Check sheet for the modelled part. Datum: model origin and axes. Units: mm. A direction names the side the tool comes from. Round coordinates to 2 decimals unless told otherwise and drop trailing zeros. Order: outer loops, then holes, each group sorted by start corner. A loop starts at its lowest first (then second) coordinate and runs counter-clockwise, first axis right, second up.
Q1. Scan lines: probe 1 along X at (y, z) = (-9, -7.5); probe 2 along Z at (x, y) = (69, 0); probe 3 along X at (y, z) = (-3.5, -5.5). Record each from-to range of solid material in increasing order.
Q2. Cross-section at A-A on x = -5. Record the cut outline in (y, z) (3 decimals), then the cut area to 3 significant figures.
Q3. Depth check by flat-ended pin: P1, Ø8.5, axis at x = -6.65, z = 0, coming from the +Y side (3 decimals); P2, Ø1.1, axis at y = 2, z = 13.5, coming from the -X side; P3, Ø1.5, axis at y = -4.5, z = -10.5, coming from the +X side; P4, Ø12, axis at y = 6, z = 7.5, coming from the +X side. Enter the tip coordinate at first touch or a pass-through.
Q4. Mould release check, pull along Y, two halves, no side actions. Record for faces 1 (the flat face through (70, 5.08, 7)), 2 (the cylindrical face through (68.61, 0.07, 10.11)), 3 (the cylindrical face through (61.14, 0.51, -12.69)): +Y half, -Y half, draft (parallel to the pull), parting line (faces both ways), or undercut.
Q5. Set-up check for faces 4 (the flat face through (33, 3.175, 10)), 5 (the cylindrical face through (70.05, -0.11, -5.08)), 6 (the flat face through (8, -3.175, 12.5)), 7 (the flat face through (33, 0, 10.16)): record each of +Z, -Z, +X, -X, +Y, -Y from which the full face is reachable in a straight line by a thin tool's end or side.
Q6. Cross-section at B-B on x = 57.5. Record the cut outline in (y, z) (3 decimals), then the cut area to 3 significant figures.
from build123d import *

# Parameters (mm, degrees)
F0_R     = 3.175
F2_DEPTH = 3.175
F3_R     = 1.524
F4_DEPTH = 7.62
F5_R     = 1.524
F6_DEPTH = 17.78
F7_R     = 1.524
F8_DEPTH = 10.414


with BuildPart() as f1:
    # F0 (on Front) → F1 (revolve)
    with BuildSketch(Plane.XZ):
        with BuildLine():
            Line((0, 15.238884), (0, 0))
            Line((0, 0), (7.112, 0))
            Line((7.112, 0), (66.294, 0))
            Line((66.294, 0), (66.294, 12.7))
            Line((66.294, 12.7), (56.134, 12.7))
            Line((56.134, 12.7), (56.134, 11.43))
            ThreePointArc((56.134, 11.43), (55.762026, 10.531974), (54.864, 10.16))
            Line((54.864, 10.16), (11.43, 10.16))
            ThreePointArc((11.43, 10.16), (10.531974, 10.531974), (10.16, 11.43))
            Line((10.16, 11.43), (10.16, 12.7))
            Line((10.16, 12.7), (7.112, 12.7))
            ThreePointArc((7.112, 12.7), (6.213974, 13.071974), (5.842, 13.97))
            Line((5.842, 13.97), (5.842, 15.24))
            Line((5.842, 15.24), (0.053232, 15.24))
            ThreePointArc((0.053232, 15.24), (0.02661, 15.239721), (0, 15.238884))
        make_face()
    revolve(axis=Axis((36.703, 0, 0), (-1, 0, 0)))

    # F0 (on Front) → F2 (join, symmetric)
    with BuildSketch(Plane.XZ):
        with BuildLine():
            Line((-0.9398, 0), (0, 0))
            Line((0, 0), (0, 15.238884))
            ThreePointArc((0, 15.238884), (-0.484346, 15.120613), (-0.885841, 14.82501))
            Line((-0.885841, 14.82501), (-10.88063, 3.847543))
            ThreePointArc((-10.88063, 3.847543), (-4.591961, 5.329721), (-0.9398, 0))
        make_face()
        with BuildLine():
            Line((0, 15.238884), (0, 0))
            Line((0, 0), (7.112, 0))
            Line((7.112, 0), (66.294, 0))
            Line((66.294, 0), (66.294, 12.7))
            Line((66.294, 12.7), (56.134, 12.7))
            Line((56.134, 12.7), (56.134, 11.43))
            ThreePointArc((56.134, 11.43), (55.762026, 10.531974), (54.864, 10.16))
            Line((54.864, 10.16), (11.43, 10.16))
            ThreePointArc((11.43, 10.16), (10.531974, 10.531974), (10.16, 11.43))
            Line((10.16, 11.43), (10.16, 12.7))
            Line((10.16, 12.7), (7.112, 12.7))
            ThreePointArc((7.112, 12.7), (6.213974, 13.071974), (5.842, 13.97))
            Line((5.842, 13.97), (5.842, 15.24))
            Line((5.842, 15.24), (0.053232, 15.24))
            ThreePointArc((0.053232, 15.24), (0.02661, 15.239721), (0, 15.238884))
        make_face()
        with BuildLine():
            Line((7.112, 0), (0, 0))
            Line((0, 0), (-0.9398, 0))
            ThreePointArc((-0.9398, 0), (-3.195791, -4.549339), (-8.182663, -5.506983))
            Line((-8.182663, -5.506983), (4.232475, -8.951452))
            ThreePointArc((4.232475, -8.951452), (5.340669, -8.738642), (5.842, -7.727678))
            Line((5.842, -7.727678), (5.842, -1.27))
            ThreePointArc((5.842, -1.27), (6.213974, -0.371974), (7.112, 0))
        make_face()
        with BuildLine():
            ThreePointArc((-8.182663, -5.506983), (-3.195791, -4.549339), (-0.9398, 0))
            ThreePointArc((-0.9398, 0), (-4.591961, 5.329721), (-10.88063, 3.847543))
            ThreePointArc((-10.88063, 3.847543), (-12.145978, -1.583727), (-8.182663, -5.506983))
        make_face()
        with Locations((-6.6548, 0)):
            Circle(F0_R, mode=Mode.SUBTRACT)
    extrude(amount=F2_DEPTH, both=True)

    # F3 (on face) → F4 (join)
    with BuildSketch(Plane.YZ.offset(66.294)):
        with BuildLine():
            ThreePointArc((-5.08, 0), (0, -5.08), (5.08, 0))
            ThreePointArc((5.08, 0), (0, 5.08), (-5.08, 0))
        make_face()
        Circle(F3_R, mode=Mode.SUBTRACT)
        with BuildLine():
            ThreePointArc((-5.08, 0), (0, 5.08), (5.08, 0))
            Line((5.08, 0), (5.08, 13.97))
            ThreePointArc((5.08, 13.97), (4.708026, 14.868026), (3.81, 15.24))
            Line((3.81, 15.24), (-3.81, 15.24))
            ThreePointArc((-3.81, 15.24), (-4.708026, 14.868026), (-5.08, 13.97))
            Line((-5.08, 13.97), (-5.08, 0))
        make_face()
    extrude(amount=F4_DEPTH)

    # F5 (on face) → F6 (cut)
    with BuildSketch(Plane.XY.offset(15.24)):
        with Locations((2.65662, 0)):
            Circle(F5_R)
    extrude(amount=-F6_DEPTH, mode=Mode.SUBTRACT)

    # F7 (on face) → F8 (cut)
    with BuildSketch(Plane.XY.offset(15.24)):
        with Locations((70.133381, 0)):
            Circle(F7_R)
    extrude(amount=-F8_DEPTH, mode=Mode.SUBTRACT)


solid = f1.part
Results found:
1. probe 1: x = 0 to 10.16, 56.13 to 66.29
1. probe 2: z = -5.08 to -1.52, 1.52 to 4.83
1. probe 3: x = 0 to 66.29
2. outline: (-3.175, -6.39) - (3.175, -6.39) - (3.175, -2.71) - (-3.175, -2.71) - close; (-3.175, 2.71) - (3.175, 2.71) - (3.175, 10.306) - (-3.175, 10.306) - close
2. area: 71.6 mm2
3. P1: stops at y = 3.175
3. P2: stops at x = -2.59
3. P3: stops at x = 66.29
3. P4: stops at x = 73.91
4. face 1: +Y half
4. face 2: undercut
4. face 3: parting line
5. face 4: +Z, +Y
5. face 5: -Z, +X
5. face 6: +Z, -Y
5. face 7: +Z, +Y, -Y
6. outline: (-3.175, 12.297) arc R12.7 ccw (long way) to (3.175, 12.297) - (3.175, 12.7) - (-3.175, 12.7) - close
6. area: 508 mm2
